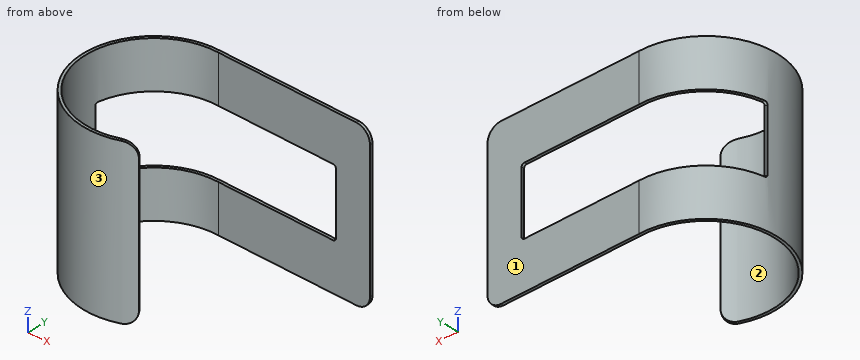
```python
from build123d import *

# Parameters (mm, degrees)
EXTRUDE_THIN1_DEPTH = 76.2
FILLET1_R           = 12.7
SKETCH2_W           = 190.5
SKETCH2_H           = 63.5
CUT_EXTRUDE1_DEPTH  = 57.15
FILLET2_R           = 2.54


with BuildPart() as part:
    # Sketch1 → Extrude-Thin1 (new, symmetric)
    with BuildSketch(Plane.XY):
        with BuildLine():
            Line((134.168540946, 66.648854011), (-7.118959054, 66.648854011))
            ThreePointArc((-7.118959054, 66.648854011), (-73.147095727, -18.135899971), (27.495287719, -55.809232643))
            Line((27.495287719, -55.809232643), (26.105523948, -53.683166638))
            ThreePointArc((26.105523948, -53.683166638), (-70.707652233, -17.428059655), (-7.154874368, 64.108854011))
            Line((-7.154874368, 64.108854011), (134.168540946, 64.108854011))
            Line((134.168540946, 64.108854011), (134.168540946, 66.648854011))
        make_face()
    extrude(amount=EXTRUDE_THIN1_DEPTH, both=True)

    # Fillet1
    fillet1_edges = [part.edges().sort_by_distance(p)[0] for p in [
        (134.168540946, 65.378854011, 76.2),
        (134.168540946, 65.378854011, -76.2),
        (26.800405833, -54.74619964, -76.2),
        (26.800405833, -54.74619964, 76.2),
    ]]
    fillet(fillet1_edges, radius=FILLET1_R)

    # Sketch2 → Cut-Extrude1 (cut, symmetric)
    with BuildSketch(Plane(origin=(0, 66.648854011, 0), x_dir=(1, 0, 0), z_dir=(0, 1, 0))):
        with Locations((7.168540946, 0)):
            Rectangle(SKETCH2_W, SKETCH2_H)
    extrude(amount=CUT_EXTRUDE1_DEPTH, both=True, mode=Mode.SUBTRACT)

    # Fillet2
    fillet2_edges = [part.edges().sort_by_distance(p)[0] for p in [
        (102.418540946, 65.378854011, -31.75),
        (102.418540946, 65.378854011, 31.75),
        (-73.697301111, 9.498854011, 31.75),
        (-73.697301111, 9.498854011, -31.75),
    ]]
    fillet(fillet2_edges, radius=FILLET2_R)


solid = part.part
```
CAD build for the part. Positions are in the model's coordinates, mm. Face numbers are marked on the shaded views. Give positions to 0.01 mm unless a question says otherwise; leave off trailing zeros. Loops run counter-clockwise (first coordinate to the right, second up) from the corner with the lowest first, then second, coordinate; pieces in that order, holes last. Notation, with made-up numbers: (-21, -38.75) -> (-14, -38.75) arc R33 cw to (-14, -2.75) -> close; hole circle Ø7 at (-11.75, 80). An arc over 180 degrees is marked (long way). Use a Markdown table: item, result.
1. Slice it at D-D (y = 0). List the corners of the cut face in (x, z).
Check result:
| item | result |
|---|---|
| outline | (-75.66, -76.2) -> (-73.12, -76.2) -> (-73.12, 76.2) -> (-75.66, 76.2) -> close |
2. Flat gauge pins, fed straight in: pin 1 (1 mm diameter, centred on y = 16.5, z = -37, fed in from -X); pin 2 (3 mm diameter, centred on x = -73.5, z = 5, fed in from +Y); pin 3 (3 mm diameter, centred on y = 66, z = 8.5, fed in from -X). Where does each tip first touch, or does it go through?
Check result:
| item | result |
|---|---|
| pin 1 | stops at x = -73.71 |
| pin 2 | stops at y = 9.5 |
| pin 3 | stops at x = 102.42 |
3. Slice it at C-C (x = 6). List the corners of the cut face in (y, z), plus the area to 3 significant figures.
Check result:
| item | result |
|---|---|
| outline | (-64.97, -76.2) -> (-62.36, -76.2) -> (-62.36, 76.2) -> (-64.97, 76.2) -> close; (64.11, -76.2) -> (66.65, -76.2) -> (66.65, -31.75) -> (64.11, -31.75) -> close; (64.11, 31.75) -> (66.65, 31.75) -> (66.65, 76.2) -> (64.11, 76.2) -> close |
| area | 623 mm^2 |
4. Wall check: L1, parallel to X at y = 0, z = 11; L2, parallel to Y at x = 17, z = 55; L3, parallel to Y at x = 100, z = 36.5. Give the ranges that are in metal, low to high. Write a range as [from, to].
Check result:
| item | result |
|---|---|
| L1 | x = [-75.66, -73.12] |
| L2 | y = [-61.4, -58.63], [64.11, 66.65] |
| L3 | y = [64.11, 66.65] |
5. Mould opens along X. For the marked faces 1, 2 and 3 say: pulls with the +X half, pulls with the -X half, needs draft (parallel to the pull), parting line crosses it, or undercut.
Check result:
| item | result |
|---|---|
| face 1 | needs draft |
| face 2 | undercut |
| face 3 | parting line crosses it |
6. Slice it at B-B (z = 17.5). List the corners of the cut face in (x, y) (3 decimals).
Check result:
| item | result |
|---|---|
| outline | (-74.981, 9.499) arc R66.675 ccw to (27.495, -55.809) -> (26.106, -53.683) arc R64.135 cw to (-72.414, 9.499) -> close; (102.419, 64.109) -> (134.169, 64.109) -> (134.169, 66.649) -> (102.419, 66.649) -> close |
7. Slice it at A-A (x = 88.5). List the corners of the cut face in (y, z).
Check result:
| item | result |
|---|---|
| outline | (64.11, -76.2) -> (66.65, -76.2) -> (66.65, -31.75) -> (64.11, -31.75) -> close; (64.11, 31.75) -> (66.65, 31.75) -> (66.65, 76.2) -> (64.11, 76.2) -> close |
